from build123d import *

# Parameters (mm, degrees)
F1_DEPTH = 25.4


with BuildPart() as f1:
    # F0 (on Top) → F1 (new body)
    with BuildSketch(Plane.XY):
        Polygon((-4.628678, 56.017287), (-46.759091, 56.110911), (-46.759091, -23.993554), (38.257439, -23.993554), (38.257439, 55.921983), align=None)
        Polygon((-70.588064, 69.903373), (-46.759091, 56.110911), (-4.628678, 56.017287), (38.257439, 55.921983), (0, 75.192399), align=None)
        Polygon((-46.759091, 59.95094), (-60.361739, 67.824297), (-1.792516, 72.924256), (24.276726, 59.79308), align=None, mode=Mode.SUBTRACT)
        Polygon((-46.759091, -23.993554), (-46.759091, 56.110911), (-70.588064, 69.903373), (-70.752643, -4.156364), align=None)
    extrude(amount=F1_DEPTH)


solid = f1.part
CAD build for the part. Positions are in the model's coordinates, mm. A direction names the side the tool comes from. Give positions to 0.01 mm unless a question says otherwise; leave off trailing zeros. Loops run counter-clockwise (first coordinate to the right, second up) from the corner with the lowest first, then second, coordinate; pieces in that order, holes last. Notation, with made-up numbers: M 70,-25.75 L 121,-25.75 A25 ccw 121,-13.75 Z; hole C -21.5,3 d7. An arc over 180 degrees is marked long. One line per question, with ' | ' between items. Start each with the question number.
1. Two-plate mould, pull along X, no slides. Class faces 1 (the face through (-53.465, 63.833, 12.522)), 2 (the face through (19.4, 65.42, 12.52)), 3 (the face through (-31.49, 70.34, 12.52)), 4 (the face through (-58.92, -13.94, 12.52)): pulls with the +X half, pulls with the -X half, needs draft (parallel to the pull), parting line crosses it, or undercut.
2. Saw through at C-C on y = 62.5. Give the cut face in (x, z).
3. Saw through at B-B on x = -21. Give the cut face in (y, z), plus the area to 3 significant figures.
4. Probe L1, parallel to X at y = 7, z = 8.25; L2, parallel to Y at x = 16, z = 23; L3, parallel to Y at x = 14.5, z = 13. List the from-to ranges inside material, lowest first. Write a range as from..to.
5. Saw through at A-A on z = 20.75. Give the cut face in (x, y).
6. Flat gauge pins, fed straight in: pin 1 (1.5 mm diameter, centred on x = -12.5, z = 12.5, fed in from +Y); pin 2 (10 mm diameter, centred on x = -21.5, z = 9.5, fed in from +Y); pin 3 (10 mm diameter, centred on y = -11, z = 18, fed in from -X). Where does each tip first touch, or does it go through?
7. 3-axis set-ups, long thin cutter, end or side, ignore diameter. For faces 5 (the face through (11.06, 66.45, 12.52)), 6 (the face through (-5, -23.994, 13)): which of +Z, -Z, +X, -X, +Y, -Y reach the whole face in a straight line?
8. Saw through at D-D on x = 28.5. Give the cut face in (y, z).
Result sheet:
1) face 1: undercut | face 2: pulls with the +X half | face 3: undercut | face 4: pulls with the -X half
2) outline: M -70.6,0 L -51.16,0 L -51.16,25.4 L -70.6,25.4 Z; M 18.9,0 L 25.2,0 L 25.2,25.4 L 18.9,25.4 Z
3) outline: M -23.99,0 L 59.89,0 L 59.89,25.4 L -23.99,25.4 Z; M 71.25,0 L 73.62,0 L 73.62,25.4 L 71.25,25.4 Z | area: 2,190 mm^2
4) L1: x = -70.73..38.26 | L2: y = -23.99..59.81, 63.96..67.13 | L3: y = -23.99..59.81, 64.72..67.89
5) outline: M -70.75,-4.16 L -46.76,-23.99 L 38.26,-23.99 L 38.26,55.92 L 0,75.19 L -70.59,69.9 Z; hole M -60.36,67.82 L -46.76,59.95 L 24.28,59.79 L -1.79,72.92 Z
6) pin 1: stops at y = 74.31 | pin 2: stops at y = 73.96 | pin 3: stops at x = -68.52
7) face 5: +Z, -Z | face 6: +Z, -Z, +X, -X, -Y
8) outline: M -23.99,0 L 60.84,0 L 60.84,25.4 L -23.99,25.4 Z
